from build123d import *

# Parameters (mm, degrees)
BOSS_EXTRUDE1_DEPTH = 76.2
CUT_EXTRUDE3_DEPTH  = 129.420802443


with BuildPart() as part:
    # Sketch1 → Boss-Extrude1 (new body)
    with BuildSketch(Plane(origin=(0, 0, 0), x_dir=(0, 0, -1), z_dir=(1, 0, 0))):
        Polygon((-6.35, 76.2), (69.85, 76.2), (69.85, 69.85), (0, 69.85), (0, 0), (-6.35, 0), align=None)
    extrude(amount=BOSS_EXTRUDE1_DEPTH)

    # Sketch7 → Cut-Extrude3 (cut, through all)
    with BuildSketch(Plane(origin=(0, 0, 0), x_dir=(-1, 0, 0), z_dir=(0, 0, -1))):
        with BuildLine():
            Line((-69.85, 67.31), (-6.35, 67.31))
            ThreePointArc((-6.35, 67.31), (-3.96875, 64.92875), (-6.35, 62.5475))
            Line((-6.35, 62.5475), (-69.85, 62.5475))
            ThreePointArc((-69.85, 62.5475), (-72.23125, 64.92875), (-69.85, 67.31))
        make_face()
    extrude(amount=-CUT_EXTRUDE3_DEPTH, mode=Mode.SUBTRACT)


solid = part.part
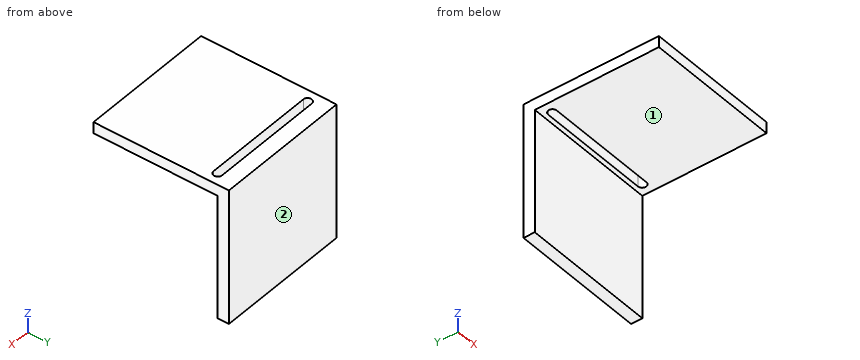
Part model, mm, in its own coordinate system. Face numbers are marked on the shaded views. A direction names the side the tool comes from. Coordinates: 2 decimals unless noted, no trailing zeros. Order: outer loops, then holes, each group sorted by start corner. A loop starts at its lowest first (then second) coordinate and runs counter-clockwise, first axis right, second up.
(1) Slice it at C-C, the plane y = 50. Write the cut outline in (x, z), and give its area (3 significant figures).
Check sheet entries:
outline: (0, 0) - (76.2, 0) - (76.2, 6.35) - (0, 6.35) - close
area: 484 mm2
(2) Pin check, flat tips, straight feed: pin 1 Ø10 at (x, y) = (48.5, 52) entering from -Z; pin 2 Ø3 at (x, z) = (13, -40) entering from -Y; pin 3 Ø5 at (x, z) = (28, 2) entering from -Y. Stop position of each tip, or through.
Check sheet entries:
pin 1: stops at z = 0
pin 2: stops at y = 69.85
pin 3: stops at y = 0
(3) Slice it at D-D, the plane z = -31. Write the cut outline in (x, y).
Check sheet entries:
outline: (0, 69.85) - (76.2, 69.85) - (76.2, 76.2) - (0, 76.2) - close
(4) Probe L1, parallel to Z at x = 14.5, y = 68.5; L2, parallel to Y at x = 14, z = -3; L3, parallel to Y at x = 6, z = 3. List the from-to ranges inside material, lowest first.
Check sheet entries:
L1: z = 0 to 6.35
L2: y = 69.85 to 76.2
L3: y = 0 to 62.57, 67.28 to 76.2
(5) Slice it at A-A, the plane z = 2. Write the cut outline in (x, y).
Check sheet entries:
outline: (0, 0) - (76.2, 0) - (76.2, 76.2) - (0, 76.2) - close; hole (6.35, 62.55) - (69.85, 62.55) arc R2.38 ccw to (69.85, 67.31) - (6.35, 67.31) arc R2.38 ccw to start
(6) Tool access for the marked faces 1 and 2: list every direction of +Z, -Z, +X, -X, +Y, -Y with a clear straight run to the whole face (end or side of a thin tool).
Check sheet entries:
face 1: -Z, +X, -X, -Y
face 2: +Z, -Z, +X, -X, +Y
(7) Slice it at B-B, the plane x = 24.5. Write the cut outline in (y, z).
Check sheet entries:
outline: (0, 0) - (62.55, 0) - (62.55, 6.35) - (0, 6.35) - close; (67.31, 0) - (69.85, 0) - (69.85, -69.85) - (76.2, -69.85) - (76.2, 6.35) - (67.31, 6.35) - close
